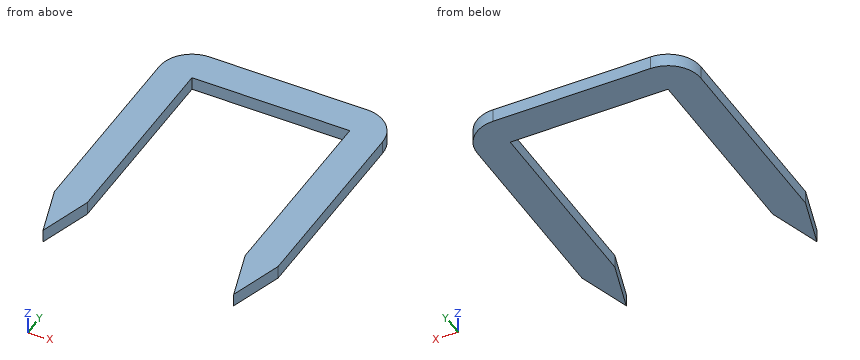
```python
from build123d import *

# Parameters (mm, degrees)
F1_DEPTH = 2


with BuildPart() as f1:
    # F0 (on Top) → F1 (new body)
    with BuildSketch(Plane.XY):
        with BuildLine():
            Line((-11.243236, 9.986477), (-11.243236, -20.013523))
            Line((-11.243236, -20.013523), (-8.743236, -28.013523))
            Line((-8.743236, -28.013523), (-6.243236, -20.013523))
            Line((-6.243236, -20.013523), (-6.243236, 9.986477))
            Line((-6.243236, 9.986477), (17.756764, 9.986477))
            Line((17.756764, 9.986477), (17.756764, -20.013523))
            Line((17.756764, -20.013523), (20.256763, -28.013523))
            Line((20.256763, -28.013523), (22.756764, -20.013523))
            Line((22.756764, -20.013523), (22.756764, 9.986477))
            ThreePointArc((22.756764, 9.986477), (21.292298, 13.522011), (17.756764, 14.986477))
            Line((17.756764, 14.986477), (-6.243236, 14.986477))
            ThreePointArc((-6.243236, 14.986477), (-9.77877, 13.522011), (-11.243236, 9.986477))
        make_face()
    extrude(amount=F1_DEPTH)


solid = f1.part
```
Verification items for the finished model (mm, model axes). Round coordinates to 2 decimals unless told otherwise and drop trailing zeros. Write each loop counter-clockwise with the first axis right and the second up, starting at its lowest first coordinate (ties: lowest second). Pieces come first, ordered by that corner, then holes. Notation, with made-up numbers: (25.5, -18) -> (60.5, -18) arc R25 ccw to (60.5, 13) -> close; hole circle Ø9 at (27, 27). An arc over 180 degrees is marked (long way). Write each question's results on one line, items separated by ' | '.
Q1. Sectioned sample at D-D, the plane y = -24. Record the boundary of the cut face in (x, z).
Derived:
outline: (-10, 0) -> (-7.49, 0) -> (-7.49, 2) -> (-10, 2) -> close; (19, 0) -> (21.51, 0) -> (21.51, 2) -> (19, 2) -> close
Q2. Sectioned sample at B-B, the plane z = 1. Record the boundary of the cut face in (x, y), and give its area (3 significant figures).
Derived:
outline: (-11.24, -20.01) -> (-8.74, -28.01) -> (-6.24, -20.01) -> (-6.24, 9.99) -> (17.76, 9.99) -> (17.76, -20.01) -> (20.26, -28.01) -> (22.76, -20.01) -> (22.76, 9.99) arc R5 ccw to (17.76, 14.99) -> (-6.24, 14.99) arc R5 ccw to (-11.24, 9.99) -> close | area: 499 mm²
Q3. Sectioned sample at C-C, the plane x = 7. Record the boundary of the cut face in (y, z).
Derived:
outline: (9.99, 0) -> (14.99, 0) -> (14.99, 2) -> (9.99, 2) -> close
Q4. Sectioned sample at A-A, the plane y = 5.5. Record the boundary of the cut face in (x, z).
Derived:
outline: (-11.24, 0) -> (-6.24, 0) -> (-6.24, 2) -> (-11.24, 2) -> close; (17.76, 0) -> (22.76, 0) -> (22.76, 2) -> (17.76, 2) -> close
Q5. Thickness scan on probe 1 along X at (y, z) = (-2, 0.85); probe 2 along Y at (x, z) = (5, 0.2); probe 3 along X at (y, z) = (-25, 1.7). Record the ranges inside material, lowest first.
Derived:
probe 1: x = -11.24 to -6.24, 17.76 to 22.76 | probe 2: y = 9.99 to 14.99 | probe 3: x = -9.68 to -7.8, 19.32 to 21.2
Q6. Go/stop test with flat-tipped pins: pin 1 Ø1 at (y, z) = (-21, 1.5) entering from +X; pin 2 Ø0.6 at (x, z) = (8, 1) entering from -Y. Record where each tip stops, or that it passes through.
Derived:
pin 1: stops at x = 22.6 | pin 2: stops at y = 9.99
